Design review of the part built by this model. Coordinates are the model's own, in mm. A direction names the side the tool comes from. Coordinates: 2 decimals unless noted, no trailing zeros. Order: outer loops, then holes, each group sorted by start corner. A loop starts at its lowest first (then second) coordinate and runs counter-clockwise, first axis right, second up. Notation, with made-up numbers: (12, 60) - (56, 60) arc R19 ccw to (56, 87) - close; hole circle Ø6 at (33, -31). An arc over 180 degrees is marked (long way). Write each question's results on one line, items separated by ' | '. Start each with the question number.
```python
from build123d import *

# Parameters (mm, degrees)
SKETCH_1_W          = 200
SKETCH_1_H          = 30
EXTRUDE_1_DEPTH     = 11
SKETCH_4_W          = 15
SKETCH_4_H          = 3
EXTRUDE_2_DEPTH     = 25
CUT_EXTRUDE_2_DEPTH = 204.776838723
CUT_EXTRUDE_3_DEPTH = 203.358592602
SKETCH_9_W          = 30
SKETCH_9_H          = 6
EXTRUDE_3_DEPTH     = 25
CUT_EXTRUDE_4_DEPTH = 203.358592602


with BuildPart() as part:
    # 草圖1 → 填料-伸長1 (new body)
    with BuildSketch(Plane.XY):
        with Locations((100, 15)):
            Rectangle(SKETCH_1_W, SKETCH_1_H)
    extrude(amount=EXTRUDE_1_DEPTH)

    # 草圖4 → 填料-伸長2 (add)
    with BuildSketch(Plane(origin=(0, 0, 0), x_dir=(-1, 0, 0), z_dir=(0, 0, -1))):
        with Locations((-107.5, 13.5)):
            Rectangle(SKETCH_4_W, SKETCH_4_H)
        with Locations((-107.5, 16.5)):
            Rectangle(SKETCH_4_W, SKETCH_4_H)
        with Locations((-92.5, 16.5)):
            Rectangle(SKETCH_4_W, SKETCH_4_H)
        with Locations((-92.5, 13.5)):
            Rectangle(SKETCH_4_W, SKETCH_4_H)
    extrude(amount=EXTRUDE_2_DEPTH)

    # 草圖5 → 除料-伸長2 (cut, through all)
    with BuildSketch(Plane(origin=(200, 0, 0), x_dir=(0, 0, -1), z_dir=(1, 0, 0))):
        Polygon((-11, 15), (-7, 15), (-7, 18.6), (-11, 19.25), align=None)
        Polygon((-7, 11.402039536), (-7, 15), (-11, 15), (-11, 10.75), align=None)
    extrude(amount=-CUT_EXTRUDE_2_DEPTH, mode=Mode.SUBTRACT)

    # 草圖6 → 除料-伸長3 (cut, through all)
    with BuildSketch(Plane.XZ.offset(-12)):
        with BuildLine():
            ThreePointArc((101.45, -12.5), (101.025304833, -11.474695167), (100, -11.05))
            Line((100, -11.05), (100, -12.5))
            Line((100, -12.5), (101.45, -12.5))
        make_face()
        with BuildLine():
            Line((100, -12.5), (100, -11.05))
            ThreePointArc((100, -11.05), (98.974695167, -11.474695167), (98.55, -12.5))
            Line((98.55, -12.5), (100, -12.5))
        make_face()
        with BuildLine():
            Line((101.45, -12.5), (100, -12.5))
            Line((100, -12.5), (100, -13.95))
            ThreePointArc((100, -13.95), (101.025304833, -13.525304833), (101.45, -12.5))
        make_face()
        with BuildLine():
            Line((100, -13.95), (100, -12.5))
            Line((100, -12.5), (98.55, -12.5))
            ThreePointArc((98.55, -12.5), (98.974695167, -13.525304833), (100, -13.95))
        make_face()
    extrude(amount=-CUT_EXTRUDE_3_DEPTH, mode=Mode.SUBTRACT)

    # 草圖9 → 填料-伸長3 (add)
    with BuildSketch(Plane(origin=(0, 0, 0), x_dir=(-1, 0, 0), z_dir=(0, 0, -1))):
        with Locations((-179.638936631, 15)):
            Rectangle(SKETCH_9_W, SKETCH_9_H)
    extrude(amount=EXTRUDE_3_DEPTH)

    # 草圖10 → 除料-伸長4 (cut, through all)
    with BuildSketch(Plane(origin=(0, 18, 0), x_dir=(1, 0, 0), z_dir=(0, 1, 0))):
        with BuildLine():
            ThreePointArc((178.188936631, 12.5), (179.638936631, 11.05), (181.088936631, 12.5))
            Line((181.088936631, 12.5), (178.188936631, 12.5))
        make_face()
        with BuildLine():
            Line((178.188936631, 12.5), (181.088936631, 12.5))
            ThreePointArc((181.088936631, 12.5), (179.638936631, 13.95), (178.188936631, 12.5))
        make_face()
    extrude(amount=-CUT_EXTRUDE_4_DEPTH, mode=Mode.SUBTRACT)


solid = part.part
```
(1) Take a section at A-A (z = -6). State the section outline as (x, y) points.
(2) Take a section at C-C (y = 3). State the section outline as (x, z) points, plus the area to 3 significant figures.
(3) Take a section at D-D (x = 108). State the section outline as (y, z) points.
(4) To check wall thickness, follow line 1 along X through (y, z) = (13.8, -12.5); line 2 along X through (y, z) = (13.25, -6); line 3 along Z through (x, y) = (176, 24.75). State the ranges of each line that lie inside material, in increasing order. Write a range as [from, to].
(5) Take a section at B-B (x = 30.5). State the section outline as (y, z) points.
(6) Tool access review of faces 1 (the face through (85, 15, -12)), 2 (the face through (194.639, 15, -12)), 3 (the face through (101.4, 18.92, 8.97)), 4 (the face through (100, 18, -10)): name each direction out of +Z, -Z, +X, -X, +Y, -Y from which nothing blocks a thin tool from reaching the whole face with its end or side.
(7) Clearance check with flat-ended pins moving along their axes: pin 1 (4 mm diameter, centred on x = 36, z = -3.5, fed in from -Y); pin 2 (15 mm diameter, centred on x = 58, y = 14, fed in from -Z); pin 3 (5 mm diameter, centred on x = 116.5, z = -20.5, fed in from +Y); pin 4 (5 mm diameter, centred on y = 15.5, z = -10.5, fed in from +X). State where each tip first meets the part, or that it passes through.
(8) Mouldability with a two-part tool opening along Y and no side actions: class faces 5 (the face through (200, 15, 5)), 6 (the face through (180, 12, -10)), 7 (the face through (101, 15, 7)) as +Y half, -Y half, draft (parallel to the pull), parting line (faces both ways), or undercut.
Worked out:
1) outline: (85, 12) - (115, 12) - (115, 18) - (85, 18) - close; (164.64, 12) - (194.64, 12) - (194.64, 18) - (164.64, 18) - close
2) outline: (0, 0) - (200, 0) - (200, 11) - (0, 11) - close | area: 2,200 mm^2
3) outline: (0, 0) - (12, 0) - (12, -25) - (18, -25) - (18, 0) - (30, 0) - (30, 11) - (19.25, 11) - (18.6, 7) - (11.4, 7) - (10.75, 11) - (0, 11) - close
4) line 1: [85, 98.55], [101.45, 115], [164.64, 178.19], [181.09, 194.64] | line 2: [85, 115], [164.64, 194.64] | line 3: [0, 11]
5) outline: (0, 0) - (30, 0) - (30, 11) - (19.25, 11) - (18.6, 7) - (11.4, 7) - (10.75, 11) - (0, 11) - close
6) face 1: -Z, -X, +Y, -Y | face 2: -Z, +X, +Y, -Y | face 3: +Z, +X, -X | face 4: -Z, +X, -X, +Y
7) pin 1: through | pin 2: z = 0 | pin 3: y = 18 | pin 4: x = 194.64
8) face 5: draft | face 6: -Y half | face 7: undercut
